Verification items for the finished model (mm, model axes). A direction names the side the tool comes from. Give positions to 0.01 mm unless a question says otherwise; leave off trailing zeros. Loops run counter-clockwise (first coordinate to the right, second up) from the corner with the lowest first, then second, coordinate; pieces in that order, holes last. Notation, with made-up numbers: (87, 38.5) - (94, 38.5) arc R11 ccw to (94, 43.5) - close; hole circle Ø1 at (87.25, -25.75). An arc over 180 degrees is marked (long way). One line per item, written item: value. Start each with the question number.
1. Sectioned sample at C-C (z = 10.25). Record the cut outline in (x, y).
2. Sectioned sample at A-A (x = -5.8). Record the cut outline in (y, z), plus the area to 3 significant figures.
3. Gauge pin test, flat end, axial feed: pin 1 (2 mm diameter, centred on x = 0, y = 1.5, fed in from +Z). Record the tip position at first contact, or that the pin passes through.
4. Sectioned sample at B-B (y = 3.35). Record the cut outline in (x, z).
5. Access from +Z, -Z, +X, -X, +Y, -Y to the whole of each face (thin tool, end or side, straight path). Record for faces 5 (the flat face through (-2.6, 3, 10)), 6 (the cylindrical face through (-3.25, 5.22, 9.97)), 7 (the flat face through (-1.8, 1.5, 10.2)), 8 (the flat face through (-2.6, 0.5, 10.2)).
6. Scan lines: L1, parallel to Y at x = 5.8, z = 6.75; L2, parallel to X at y = 3.25, z = 5; L3, parallel to Z at x = 0, y = 0.5. Record each from-to range of solid material in increasing order. Write a range as [from, to].
7. Sectioned sample at D-D (y = 1.5). Record the cut outline in (x, z), plus the area to 3 significant figures.
8. Mould release check, pull along Y, two halves, no side actions. Record for faces 1 (the flat face through (0, 0, 6)), 2 (the cylindrical face through (4.274, 3.831, 6.591)), 3 (the flat face through (2.6, 0.5, 10.2)), 4 (the cylindrical face through (-4.274, 3.831, 6.591)): pulls with the +Y half, pulls with the -Y half, needs draft (parallel to the pull), parting line crosses it, or undercut.
from build123d import *

# Parameters (mm, degrees)
SKETCH1_W           = 18
SKETCH1_H           = 6.7
BOSS_EXTRUDE1_DEPTH = 13
CUT_EXTRUDE1_REACH  = 19.172
SKETCH3_R           = 3.25
CUT_EXTRUDE2_DEPTH  = 3
SKETCH4_W           = 0.8
SKETCH4_H           = 1
BOSS_EXTRUDE2_DEPTH = 5.6
CUT_EXTRUDE3_REACH  = 19.172
SKETCH8_R           = 1.6


with BuildPart() as part:
    # Sketch1 → Boss-Extrude1 (new body)
    with BuildSketch(Plane.XY):
        with Locations((0, 3.35)):
            Rectangle(SKETCH1_W, SKETCH1_H)
    extrude(amount=BOSS_EXTRUDE1_DEPTH)

    # Sketch2 → Cut-Extrude1 (cut, up to next)
    with BuildSketch(Plane.XZ, mode=Mode.PRIVATE) as cut_extrude1_sk1:
        Polygon((-2.6, 12.6), (-2.6, 13), (2.6, 13), (2.6, 12.6), (2.6, 7.4), (-2.6, 7.4), align=None)
    cut_extrude1_tool1 = extrude(cut_extrude1_sk1.sketch, amount=-CUT_EXTRUDE1_REACH, mode=Mode.PRIVATE) & part.part
    add(cut_extrude1_tool1.solids().sort_by_distance((0, 0, 10.2))[0], mode=Mode.SUBTRACT)

    # Sketch3 → Cut-Extrude2 (cut)
    with BuildSketch(Plane(origin=(0, 6.7, 0), x_dir=(1, 0, 0), z_dir=(0, 1, 0))):
        with Locations((0, -10)):
            Circle(SKETCH3_R)
    extrude(amount=-CUT_EXTRUDE2_DEPTH, mode=Mode.SUBTRACT)

    # Sketch4 → Boss-Extrude2 (add)
    with BuildSketch(Plane.XY.offset(13)):
        with Locations((-2.2, 1.5)):
            Rectangle(SKETCH4_W, SKETCH4_H)
        with Locations((2.2, 1.5)):
            Rectangle(SKETCH4_W, SKETCH4_H)
    extrude(amount=-BOSS_EXTRUDE2_DEPTH)

    # Sketch8 → Cut-Extrude3 (cut, up to next)
    with BuildSketch(Plane.XY.offset(13), mode=Mode.PRIVATE) as cut_extrude3_sk1:
        with Locations((-5.8, 3.35)):
            Circle(SKETCH8_R)
    cut_extrude3_tool1 = extrude(cut_extrude3_sk1.sketch, amount=-CUT_EXTRUDE3_REACH, mode=Mode.PRIVATE) & part.part
    cut_extrude3 = cut_extrude3_tool1.solids().sort_by_distance((-5.8, 3.35, 13))[0]
    add(cut_extrude3, mode=Mode.SUBTRACT)

    # Mirror1: Cut-Extrude3 across plane
    add(cut_extrude3.mirror(Plane(origin=(0, 0, 0), x_dir=(0, 0, 1), z_dir=(1, 0, 0))), mode=Mode.SUBTRACT)


solid = part.part
Results are:
1. outline: (-9, 0) - (-2.6, 0) - (-2.6, 1) - (-1.8, 1) - (-1.8, 2) - (-2.6, 2) - (-2.6, 3.7) - (-3.24, 3.7) - (-3.24, 6.7) - (-9, 6.7) - close; (1.8, 1) - (2.6, 1) - (2.6, 0) - (9, 0) - (9, 6.7) - (3.24, 6.7) - (3.24, 3.7) - (2.6, 3.7) - (2.6, 2) - (1.8, 2) - close; hole circle Ø3.2 at (-5.8, 3.35); hole circle Ø3.2 at (5.8, 3.35)
2. outline: (0, 0) - (1.75, 0) - (1.75, 13) - (0, 13) - close; (4.95, 0) - (6.7, 0) - (6.7, 13) - (4.95, 13) - close
2. area: 45.5 mm^2
3. pin 1: stops at z = 7.4
4. outline: (-9, 0) - (-7.4, 0) - (-7.4, 13) - (-9, 13) - close; (-4.2, 0) - (4.2, 0) - (4.2, 13) - (2.6, 13) - (2.6, 7.4) - (-2.6, 7.4) - (-2.6, 13) - (-4.2, 13) - close; (7.4, 0) - (9, 0) - (9, 13) - (7.4, 13) - close
5. face 5: +Z, +Y
5. face 6: +Y
5. face 7: +Z, +Y, -Y
5. face 8: +Z, -Y
6. L1: y = [0, 1.75], [4.95, 6.7]
6. L2: x = [-9, -7.4], [-4.2, 4.2], [7.4, 9]
6. L3: z = [0, 7.4]
7. outline: (-9, 0) - (9, 0) - (9, 13) - (1.8, 13) - (1.8, 7.4) - (-1.8, 7.4) - (-1.8, 13) - (-9, 13) - close
7. area: 214 mm^2
8. face 1: pulls with the -Y half
8. face 2: undercut
8. face 3: needs draft
8. face 4: undercut
